Source: CAD feature listing. Evaluate the final solid. Frame: model axes, mm. A direction names the side the tool comes from. Coordinates: 2 decimals unless noted, no trailing zeros. Loops run counter-clockwise (first coordinate to the right, second up) from the corner with the lowest first, then second, coordinate; pieces in that order, holes last. Notation, with made-up numbers: (-37, -35.75) - (-23, -35.75) arc R12 cw to (-23, -16.75) - close; hole circle Ø1 at (-12, -27.75). An arc over 180 degrees is marked (long way). Write item = value, one per line. Start each with the question number.
from build123d import *

# Parameters (mm, degrees)
F1_DEPTH = 2.5


# Not quite as in the source:
# - ends of sketch curves that miss each other by under 0.0002 mm in the source are joined


with BuildPart() as f1:
    # F0 (on Right) → F1 (new body, symmetric)
    with BuildSketch(Plane.YZ):
        Polygon((-135, 25), (-145, 25), (-144.9999958277, 15), (-139.9999958277, 15), (-139.9999958277, 5), (-144.9999958277, 5), (-144.9999958277, -5), (-139.9999958277, -5), (-139.9999958277, -15), (-144.9999958277, -15), (-144.9999958277, -25), (-135, -25), (-135, -20), (-125, -20), (-125, -25), (-115, -25), (-115, -20), (-105, -20), (-105, -25), (-95, -25), (-95, -20), (-85, -20), (-85, -25), (-75, -25), (-75, -20), (-65, -20), (-65, -25), (-55, -25), (-55, -20), (-45, -20), (-45, -25), (-35, -25), (-35, -20), (-25, -20), (-25, -25), (-15, -25), (-15, -20), (-5, -20), (-5, -25), (5, -25), (5, -20), (15, -20), (15, -25), (25, -25), (25, -20), (35, -20), (35, -25), (45, -25), (45, -20), (55, -20), (55, -25), (65, -25), (65, -20), (75, -20), (75, -25), (85, -25), (85, -20), (95, -20), (95, -25), (105, -25), (105, -20), (115, -20), (115, -25), (125, -25), (125, -20), (135, -20), (135, -25), (145, -25), (145, -15), (140, -15), (140, -5), (145, -5), (145, 5), (140, 5), (140, 15), (145, 15), (145, 25), (135, 25), (135, 20), (125, 20), (125, 25), (115, 25), (115, 20), (105, 20), (105, 25), (95, 25), (95, 20), (85, 20), (85, 25), (75, 25), (75, 20), (65, 20), (65, 25), (55, 25), (55, 20), (45, 20), (45, 25), (35, 25), (35, 20), (25, 20), (25, 25), (15, 25), (15, 20), (5, 20), (5, 25), (-5, 25), (-5, 20), (-15, 20), (-15, 25), (-25, 25), (-25, 20), (-35, 20), (-35, 25), (-45, 25), (-45, 20), (-55, 20), (-55, 25), (-65, 25), (-65, 20), (-75, 20), (-75, 25), (-85, 25), (-85, 20), (-95, 20), (-95, 25), (-105, 25), (-105, 20), (-115, 20), (-115, 25), (-125, 25), (-125, 20), (-135, 20), align=None)
    extrude(amount=F1_DEPTH, both=True)


solid = f1.part
Item 1: Reachability of faces 1 (the flat face through (0, 15, 23)), 2 (the flat face through (0, 30, -20)), 3 (the flat face through (0, 143, 5)) from +Z, -Z, +X, -X, +Y, -Y: full face, straight path, thin tool, end or side. Return the list, or none.
Item 2: First-contact query: pin 1 (1.5 mm diameter, centred on x = 0.5, y = -112, fed in from +Z); pin 2 (1.5 mm diameter, centred on x = 1, y = 28, fed in from -Z). Flat tips, straight axial feed; report the tip coordinate or a pass-through.
Item 3: Cut plane B-B (z = 12). Return the cut outline in (x, y), then the cut area to 3 significant figures.
Item 4: Cut plane A-A (y = 68). Return the cut outline in (x, z), then the cut area to 3 significant figures.
Item 5: Material intervals for L1, parallel to Y at x = 1.3, z = -10.5; L2, parallel to Z at x = -1.35, y = -127, sorted ascending. Write a range as [from, to].
Responses:
q1.face_1 = +Z, +X, -X
q1.face_2 = -Z, +X, -X
q1.face_3 = +X, -X, +Y
q2.pin_1 = 20
q2.pin_2 = -20
q3.outline = (-2.5, -140) - (2.5, -140) - (2.5, 140) - (-2.5, 140) - close
q3.area = 1,400 mm2
q4.outline = (-2.5, -20) - (2.5, -20) - (2.5, 20) - (-2.5, 20) - close
q4.area = 200 mm2
q5.L1 = [-140, 140]
q5.L2 = [-20, 20]
